```python
from build123d import *

# Parameters (mm, degrees)
SKETCH1_W           = 200
SKETCH1_H           = 300
BOSS_EXTRUDE1_DEPTH = 3
CUT_EXTRUDE1_DEPTH  = 181.302523554


with BuildPart() as part:
    # Sketch1 → Boss-Extrude1 (new body)
    with BuildSketch(Plane(origin=(0, 0, 0), x_dir=(1, 0, 0), z_dir=(0, 1, 0))):
        Rectangle(SKETCH1_W, SKETCH1_H)
    extrude(amount=BOSS_EXTRUDE1_DEPTH)

    # Sketch3 → Cut-Extrude1 (cut, through all)
    with BuildSketch(Plane(origin=(0, 3, 0), x_dir=(1, 0, 0), z_dir=(0, 1, 0))):
        Polygon((0, 150), (50, 150), (50, 50), (-50, 50), (-50, 150), align=None)
    extrude(amount=-CUT_EXTRUDE1_DEPTH, mode=Mode.SUBTRACT)


solid = part.part
```
Verification items for the finished model (mm, model axes). Give positions to 0.01 mm unless a question says otherwise; leave off trailing zeros. Order: outer loops, then holes, each group sorted by start corner. A loop starts at its lowest first (then second) coordinate and runs counter-clockwise, first axis right, second up. Notation, with made-up numbers: (-16.5, 50.5) -> (3.5, 50.5) arc R26 cw to (3.5, 67.5) -> close; hole circle Ø2 at (24, -39.75). An arc over 180 degrees is marked (long way). Use a Markdown table: item, result.
1) Section check A-A, the plane z = -109. Record the boundary of the cut face in (x, y), then the cut area to 3 significant figures.
Results:
| item | result |
|---|---|
| outline | (-100, 0) -> (-50, 0) -> (-50, 3) -> (-100, 3) -> close; (50, 0) -> (100, 0) -> (100, 3) -> (50, 3) -> close |
| area | 300 mm² |
2) Depth check by flat-ended pin: pin 1 Ø0.9 at (x, y) = (-24.5, 2) entering from -Z. Enter the tip coordinate at first touch or a pass-through.
Results:
| item | result |
|---|---|
| pin 1 | z = -50 |
3) Material ranges on probe 1 along X at (y, z) = (2.15, -97); probe 2 along Z at (x, y) = (-39, 1.9), recorded low to high.
Results:
| item | result |
|---|---|
| probe 1 | -100 to -50, 50 to 100 |
| probe 2 | -50 to 150 |
4) Section check C-C, the plane x = -43. Record the boundary of the cut face in (y, z).
Results:
| item | result |
|---|---|
| outline | (0, -50) -> (3, -50) -> (3, 150) -> (0, 150) -> close |
5) Section check B-B, the plane y = 2.15. Record the boundary of the cut face in (x, z), then the cut area to 3 significant figures.
Results:
| item | result |
|---|---|
| outline | (-100, -150) -> (-50, -150) -> (-50, -50) -> (50, -50) -> (50, -150) -> (100, -150) -> (100, 150) -> (-100, 150) -> close |
| area | 50,000 mm² |
